from build123d import *

# Parameters (mm, degrees)
F0_R     = 1.5875
F1_DEPTH = 2.54
F2_R     = 5.08


with BuildPart() as f1:
    # F0 (on Top) → F1 (new body)
    with BuildSketch(Plane.XY):
        with BuildLine():
            Line((30.90323, 48.074035), (0, 56.374997))
            Line((0, 56.374997), (-30.90323, 48.074035))
            ThreePointArc((-30.90323, 48.074035), (-49.493352, 28.575), (-57.084951, 2.725965))
            Line((-57.084951, 2.725965), (-48.822179, -28.187498))
            Line((-48.822179, -28.187498), (-26.181721, -50.8))
            ThreePointArc((-26.181721, -50.8), (0, -57.15), (26.181721, -50.8))
            Line((26.181721, -50.8), (48.822179, -28.187498))
            Line((48.822179, -28.187498), (57.084951, 2.725965))
            ThreePointArc((57.084951, 2.725965), (49.493352, 28.575), (30.90323, 48.074035))
        make_face()
        with Locations((-43.994091, -25.4)):
            Circle(F0_R, mode=Mode.SUBTRACT)
        with Locations((0, -50.8)):
            Circle(F0_R, mode=Mode.SUBTRACT)
        with Locations((43.994091, -25.4)):
            Circle(F0_R, mode=Mode.SUBTRACT)
        with Locations((-43.994091, 25.4)):
            Circle(F0_R, mode=Mode.SUBTRACT)
        with BuildLine():
            ThreePointArc((47.625, 0), (-33.67596, -33.67596), (0, 47.625))
            ThreePointArc((0, 47.625), (33.67596, 33.67596), (47.625, 0))
        make_face(mode=Mode.SUBTRACT)
        with Locations((43.994091, 25.4)):
            Circle(F0_R, mode=Mode.SUBTRACT)
        with BuildLine():
            ThreePointArc((1.5875, 50.8), (1.122532, 49.677468), (0, 49.2125))
            ThreePointArc((0, 49.2125), (-1.5875, 50.8), (0, 52.3875))
            ThreePointArc((0, 52.3875), (1.122532, 51.922532), (1.5875, 50.8))
        make_face(mode=Mode.SUBTRACT)
        with BuildLine():
            ThreePointArc((47.625, 0), (33.67596, 33.67596), (0, 47.625))
            ThreePointArc((0, 47.625), (-33.67596, -33.67596), (47.625, 0))
        make_face()
        with BuildLine():
            ThreePointArc((19.05, 0), (-13.470384, -13.470384), (0, 19.05))
            ThreePointArc((0, 19.05), (13.470384, 13.470384), (19.05, 0))
        make_face(mode=Mode.SUBTRACT)
    extrude(amount=F1_DEPTH)

    # F2
    f2_edges = [f1.edges().sort_by_distance(p)[0] for p in [
        (-48.822179, -28.187498, 1.27),
    ]]
    fillet(f2_edges, radius=F2_R)


solid = f1.part
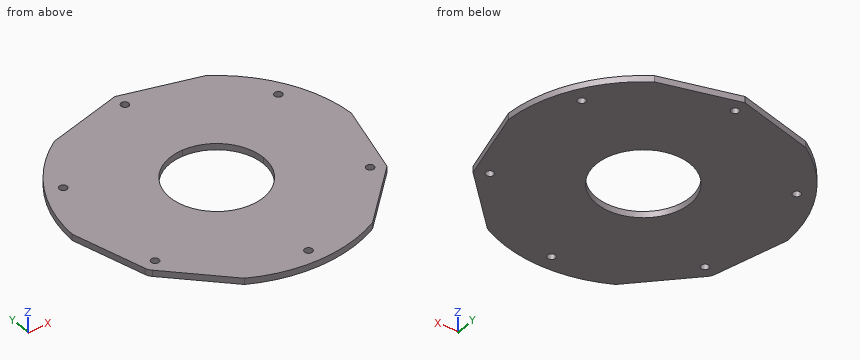
Model file for the job. Use its own axes, mm. Give positions to 0.01 mm unless a question says otherwise; leave off trailing zeros. Loops run counter-clockwise (first coordinate to the right, second up) from the corner with the lowest first, then second, coordinate; pieces in that order, holes last.
1) Saw through at D-D (y = 25.4). Write the cut outline in (x, z).
2) Saw through at A-A (x = -8.5). Write the cut outline in (y, z), plus the area to 3 significant figures.
3) Saw through at B-B (z = 1.8). Count the separate pieces of the cut face and the enclosed holes in it, plus the area to 3 significant figures.
4) Wall check: line 1 (Y direction, x = 7.5, z = 0.35); line 2 (X direction, y = -10, z = 1.3); line 3 (X direction, y = 43.5, z = 1.9). Give the ranges that are in metal, low to high.
5) Flat gauge pin, fed straight in: pin 1 Ø2.5 at (x, y) = (-43.99, 25.4) entering from -Z. Where does the tip first touch, or does it go through?
6) Saw through at C-C (x = -44). Write the cut outline in (y, z).
Answer block:
1. outline: (-51.2, 0) - (-45.58, 0) - (-45.58, 2.54) - (-51.2, 2.54) - close; (-42.41, 0) - (42.41, 0) - (42.41, 2.54) - (-42.41, 2.54) - close; (45.58, 0) - (51.2, 0) - (51.2, 2.54) - (45.58, 2.54) - close
2. outline: (-56.51, 0) - (-17.05, 0) - (-17.05, 2.54) - (-56.51, 2.54) - close; (17.05, 0) - (54.09, 0) - (54.09, 2.54) - (17.05, 2.54) - close
2. area: 194 mm2
3. separate pieces: 1
3. enclosed holes: 7
3. area: 8,700 mm2
4. line 1: y = -56.66 to -17.51, 17.51 to 54.36
4. line 2: x = -53.68 to -16.21, 16.21 to 53.68
4. line 3: x = -37.07 to 37.07
5. pin 1: passes through
6. outline: (-33, 0) - (-26.99, 0) - (-26.99, 2.54) - (-33, 2.54) - close; (-23.81, 0) - (23.81, 0) - (23.81, 2.54) - (-23.81, 2.54) - close; (26.99, 0) - (36.47, 0) - (36.47, 2.54) - (26.99, 2.54) - close
